Here's how the part is built. I have some questions about the finished solid (model axes, mm). A direction names the side the tool comes from. Coordinates: 2 decimals unless noted, no trailing zeros.
Item 1: If we mould it in two halves opening along Z, with no side actions, what happens to faces 3 (the face through (-6, -118, -10)), 4 (the face through (-10, -118, 6)), 5 (the face through (4.5, -118, 0)), 6 (the face through (-4.5, -118, 0))? For each: pulls with the +Z half, pulls with the -Z half, needs draft (parallel to the pull), parting line crosses it, or undercut.
Item 2: Please list where these lines run through material, in increasing order: line 1 (X direction, y = -86.5, z = -5.5); line 2 (X direction, y = -144, z = -8.25); line 3 (Z direction, x = 4.75, y = -186).
Item 3: I'm going to push flat-ended pins straight in: P1, Ø3.5, axis at y = -166, z = -0.5, coming from the -X side; P2, Ø0.8, axis at y = -151.5, z = -9, coming from the +X side. Where does each tip first touch, or does it pass through?
Item 4: For faces 1 (the face through (6, -118, 10)), 2 (the face through (0, -118, -4.5)), which set-ups out of +Z, -Z, +X, -X, +Y, -Y let a thin tool reach every point of the face, with its end or its side?
from build123d import *

# Parameters (mm, degrees)
F1_DEPTH = 240


with BuildPart() as f1:
    # F0 (on Front) → F1 (new body)
    with BuildSketch(Plane.XZ):
        with BuildLine():
            Line((3, -10), (8.5, -10))
            ThreePointArc((8.5, -10), (9.5606601718, -9.5606601718), (10, -8.5))
            Line((10, -8.5), (10, -3))
            Line((10, -3), (8.5, -3))
            Line((8.5, -3), (8.5, -6))
            Line((8.5, -6), (7.0606601718, -6))
            Line((7.0606601718, -6), (4.5, -3.4393398282))
            Line((4.5, -3.4393398282), (4.5, 3.4393398282))
            Line((4.5, 3.4393398282), (7.0606601718, 6))
            Line((7.0606601718, 6), (8.5, 6))
            Line((8.5, 6), (8.5, 3))
            Line((8.5, 3), (10, 3))
            Line((10, 3), (10, 8.5))
            ThreePointArc((10, 8.5), (9.5606601718, 9.5606601718), (8.5, 10))
            Line((8.5, 10), (3, 10))
            Line((3, 10), (3, 8.5))
            Line((3, 8.5), (6, 8.5))
            Line((6, 8.5), (6, 7.0606601718))
            Line((6, 7.0606601718), (3.4393398282, 4.5))
            Line((3.4393398282, 4.5), (-3.4393398282, 4.5))
            Line((-3.4393398282, 4.5), (-6, 7.0606601718))
            Line((-6, 7.0606601718), (-6, 8.5))
            Line((-6, 8.5), (-3, 8.5))
            Line((-3, 8.5), (-3, 10))
            Line((-3, 10), (-8.5, 10))
            ThreePointArc((-8.5, 10), (-9.5606601718, 9.5606601718), (-10, 8.5))
            Line((-10, 8.5), (-10, 3))
            Line((-10, 3), (-8.5, 3))
            Line((-8.5, 3), (-8.5, 6))
            Line((-8.5, 6), (-7.0606601718, 6))
            Line((-7.0606601718, 6), (-4.5, 3.4393398282))
            Line((-4.5, 3.4393398282), (-4.5, -3.4393398282))
            Line((-4.5, -3.4393398282), (-7.0606601718, -6))
            Line((-7.0606601718, -6), (-8.5, -6))
            Line((-8.5, -6), (-8.5, -3))
            Line((-8.5, -3), (-10, -3))
            Line((-10, -3), (-10, -8.5))
            ThreePointArc((-10, -8.5), (-9.5606601718, -9.5606601718), (-8.5, -10))
            Line((-8.5, -10), (-3, -10))
            Line((-3, -10), (-3, -8.5))
            Line((-3, -8.5), (-6, -8.5))
            Line((-6, -8.5), (-6, -7.0606601718))
            Line((-6, -7.0606601718), (-3.4393398282, -4.5))
            Line((-3.4393398282, -4.5), (3.4393398282, -4.5))
            Line((3.4393398282, -4.5), (6, -7.0606601718))
            Line((6, -7.0606601718), (6, -8.5))
            Line((6, -8.5), (3, -8.5))
            Line((3, -8.5), (3, -10))
        make_face()
        with BuildLine():
            ThreePointArc((-1.1560121095, 2.2166722813), (0, 2.5), (1.1560121095, 2.2166722813))
            Line((1.1560121095, 2.2166722813), (1.4393398282, 2.5))
            Line((1.4393398282, 2.5), (2.5, 1.4393398282))
            Line((2.5, 1.4393398282), (2.2166722813, 1.1560121095))
            ThreePointArc((2.2166722813, 1.1560121095), (2.5, 0), (2.2166722813, -1.1560121095))
            Line((2.2166722813, -1.1560121095), (2.5, -1.4393398282))
            Line((2.5, -1.4393398282), (1.4393398282, -2.5))
            Line((1.4393398282, -2.5), (1.1560121095, -2.2166722813))
            ThreePointArc((1.1560121095, -2.2166722813), (0, -2.5), (-1.1560121095, -2.2166722813))
            Line((-1.1560121095, -2.2166722813), (-1.4393398282, -2.5))
            Line((-1.4393398282, -2.5), (-2.5, -1.4393398282))
            Line((-2.5, -1.4393398282), (-2.2166722813, -1.1560121095))
            ThreePointArc((-2.2166722813, -1.1560121095), (-2.5, 0), (-2.2166722813, 1.1560121095))
            Line((-2.2166722813, 1.1560121095), (-2.5, 1.4393398282))
            Line((-2.5, 1.4393398282), (-1.4393398282, 2.5))
            Line((-1.4393398282, 2.5), (-1.1560121095, 2.2166722813))
        make_face(mode=Mode.SUBTRACT)
    extrude(amount=F1_DEPTH)


solid = f1.part
Answer:
1. face 3: pulls with the -Z half
1. face 4: needs draft
1. face 5: undercut
1. face 6: undercut
2. line 1: x = -10 to -8.5, -6.56 to -4.44, 4.44 to 6.56, 8.5 to 10
2. line 2: x = -10 to -6, 6 to 10
2. line 3: z = -10 to -8.5, -5.81 to -3.69, 3.69 to 5.81, 8.5 to 10
3. P1: stops at x = -4.5
3. P2: stops at x = 10
4. face 1: +Z, +X, -X, +Y, -Y
4. face 2: +Y, -Y
